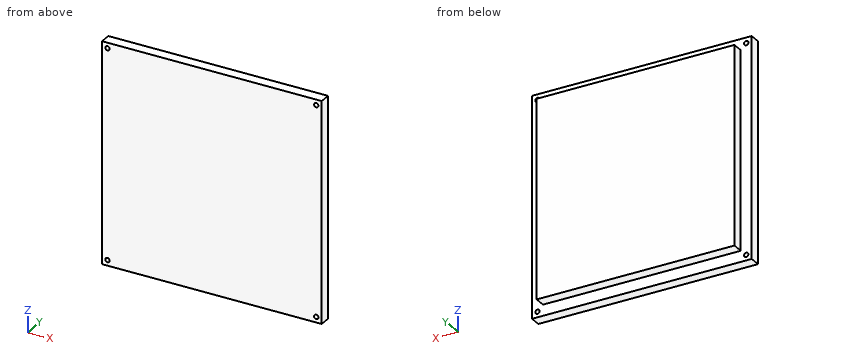
Autodesk Inventor part; units mm, degrees
ref_plane "YZ Plane" through (0, 0, 0) normal (1, 0, 0) x (0, 1, 0)
ref_plane "XZ Plane" through (0, 0, 0) normal (0, 1, 0) x (-1, 0, 0)
ref_plane "XY Plane" through (0, 0, 0) normal (0, 0, 1) x (1, 0, 0)
sketch "Sketch1" plane through (0, 0, 0) normal (0, 1, 0) x (-1, 0, 0)
  point P0 (0, 0)
sketch "Sketch2" plane through (0, 0, 0) normal (0, 1, 0) x (-1, 0, 0)
  line L0 (50, -50) -> (-50, -50)
  line L1 (-50, -50) -> (-50, 50)
  line L2 (-50, 50) -> (50, 50)
  line L3 (50, 50) -> (50, -50)
  point P0 (0, 0)
  point P1 (0, 0)
  dimension "d0" = 100
  dimension "d1" = 100
  dimension "d3" = 50
extrude "Extrusion1" add sketch "Sketch2" along normal blind 5
sketch "Sketch3" plane through (0, 5, 0) normal (0, 1, 0) x (1, 0, 0)
  circle A0 centre (-47.5, 47.5) radius 1
  line L0 (-50, 50) -> (-50, -50)
  line L1 (50, 50) -> (-50, 50)
  line L2 (50, -50) -> (50, 50)
  circle A1 centre (47.5, 47.5) radius 1
  line L3 (-50, -50) -> (50, -50)
  circle A2 centre (-47.5, -47.5) radius 1
  circle A3 centre (47.5, -47.5) radius 1
  point P0 (0, 0)
  dimension "d6" = 2.5
  dimension "d7" = 2.5
  dimension "d8" = 2
  dimension "d9" = 2.5
  dimension "d10" = 2.5
  dimension "d11" = 2.5
  dimension "d12" = 2.5
  dimension "d13" = 2.5
  dimension "d14" = 2.5
hole "Hole1" at (-47.5062, 5, -47.5057) direction (0, -1, 0) diameter 2 end through all
hole "Hole2" at (-47.4938, 5, 47.4921) direction (0, -1, 0) diameter 2 end through all
hole "Hole3" at (47.5124, 5, 47.4796) direction (0, -1, 0) diameter 2 end through all
hole "Hole4" at (47.5, 5, -47.5) direction (0, -1, 0) diameter 2 end through all
sketch "Sketch4" plane through (0, 5, 0) normal (0, 1, 0) x (1, 0, 0)
  line L0 (-45, 45) -> (45, 45)
  line L1 (45, 45) -> (45, -45)
  line L2 (45, -45) -> (-45, -45)
  line L3 (-45, -45) -> (-45, 45)
  line L4 (50, 50) -> (50, -50)
  line L5 (50, 50) -> (-50, 50)
  line L6 (-50, 50) -> (-50, -50)
  line L7 (-50, -50) -> (50, -50)
  point P0 (0, 0)
  dimension "d49" = 5
  dimension "d50" = 5
  dimension "d51" = 5
  dimension "d52" = 5
extrude "Extrusion2" add sketch "Sketch4" along normal blind 5 contours L0 L1 L2 L3
properties part number "cubesat_top"
Check sheet for the modelled part. Datum: model origin and axes. Units: mm. Coordinates: 2 decimals unless noted, no trailing zeros. Write each loop counter-clockwise with the first axis right and the second up, starting at its lowest first coordinate (ties: lowest second). Pieces come first, ordered by that corner, then holes. Notation, with made-up numbers: (9.5, 28.5) -> (51.5, 28.5) arc R18 cw to (51.5, 57.5) -> close; hole circle Ø8 at (64, 8). An arc over 180 degrees is marked (long way). Use a Markdown table: item, result.
1. Sectioned sample at B-B (x = -28.5). Enter the section's corners in (y, z), plus the area to 3 significant figures.
Reported:
| item | result |
|---|---|
| outline | (0, -50) -> (5, -50) -> (5, -45) -> (10, -45) -> (10, 45) -> (5, 45) -> (5, 50) -> (0, 50) -> close |
| area | 950 mm2 |
2. Scan lines: line 1 along X through (y, z) = (1.8, -47.5); line 2 along Z through (x, y) = (47.5, 3.45); line 3 along Z through (x, y) = (12.5, 6.5). Record each from-to range of solid material in increasing order.
Reported:
| item | result |
|---|---|
| line 1 | x = -50 to -48.51, -46.51 to 46.5, 48.5 to 50 |
| line 2 | z = -50 to -48.5, -46.5 to 46.48, 48.48 to 50 |
| line 3 | z = -45 to 45 |
3. Sectioned sample at A-A (z = 7). Enter the section's corners in (x, y), plus the area to 3 significant figures.
Reported:
| item | result |
|---|---|
| outline | (-50, 0) -> (50, 0) -> (50, 5) -> (45, 5) -> (45, 10) -> (-45, 10) -> (-45, 5) -> (-50, 5) -> close |
| area | 950 mm2 |
4. Go/stop test with flat-tipped pins: pin 1 Ø1.5 at (y, z) = (7.5, -13) entering from +X; pin 2 Ø2.5 at (x, z) = (-47.51, -47.51) entering from +Y; pin 3 Ø1 at (x, y) = (22.5, 6.5) entering from +Z. Record where each tip stops, or that it passes through.
Reported:
| item | result |
|---|---|
| pin 1 | stops at x = 45 |
| pin 2 | stops at y = 5 |
| pin 3 | stops at z = 45 |
5. Sectioned sample at C-C (y = 7.5). Enter the section's corners in (x, z).
Reported:
| item | result |
|---|---|
| outline | (-45, -45) -> (45, -45) -> (45, 45) -> (-45, 45) -> close |
